```python
from build123d import *

# Parameters (mm, degrees)
BOSS_EXTRUDE1_DEPTH = 4.7
SKETCH2_R           = 8.5
BOSS_EXTRUDE2_DEPTH = 1
SKETCH4_R           = 6.5
SKETCH3_R           = 8.5
SKETCH5_R           = 4.25
BOSS_EXTRUDE3_DEPTH = 7
CHAMFER1_SIZE       = 0.4
SKETCH6_R           = 0.75
CUT_EXTRUDE1_DEPTH  = 7
CUT_EXTRUDE2_START  = -1
CUT_EXTRUDE2_DEPTH  = 1


with BuildPart() as part:
    # Sketch1 → Boss-Extrude1 (new body)
    with BuildSketch(Plane(origin=(0, 0, 0), x_dir=(1, 0, 0), z_dir=(0, 1, 0))):
        Polygon((0, 6.92820323), (6, 3.464101615), (6, -3.464101615), (0, -6.92820323), (-6, -3.464101615), (-6, 3.464101615), align=None)
    extrude(amount=BOSS_EXTRUDE1_DEPTH)

    # Sketch2 → Boss-Extrude2 (add)
    with BuildSketch(Plane(origin=(0, 4.7, 0), x_dir=(1, 0, 0), z_dir=(0, 1, 0))):
        with Locations(Location((0, 0, 0), (0, 0, 270))):
            Circle(SKETCH2_R)
    extrude(amount=BOSS_EXTRUDE2_DEPTH)

    # Sketch4 → Loft1 section 0
    with BuildSketch(Plane(origin=(0, 15.7, 0), x_dir=(1, 0, 0), z_dir=(0, 1, 0))):
        Circle(SKETCH4_R)
    # Sketch3 → Loft1 section 1
    with BuildSketch(Plane(origin=(0, 5.7, 0), x_dir=(1, 0, 0), z_dir=(0, 1, 0))):
        Circle(SKETCH3_R)
    loft()

    # Sketch5 → Boss-Extrude3 (add)
    with BuildSketch(Plane(origin=(0, 15.7, 0), x_dir=(1, 0, 0), z_dir=(0, 1, 0))):
        with Locations(Location((0, 0, 0), (0, 0, 270))):
            Circle(SKETCH5_R)
        with BuildLine():
            Line((-1.95, 2.044046232), (-1.95, -2.044046232))
            ThreePointArc((-1.95, -2.044046232), (0, -2.825), (1.95, -2.044046232))
            Line((1.95, -2.044046232), (1.95, 2.044046232))
            ThreePointArc((1.95, 2.044046232), (0, 2.825), (-1.95, 2.044046232))
        make_face(mode=Mode.SUBTRACT)
    extrude(amount=BOSS_EXTRUDE3_DEPTH)

    # Chamfer1
    chamfer1_edges = [part.edges().sort_by_distance(p)[0] for p in [
        (-6.5, 15.7, 0),
        (0, 22.7, -4.25),
        (0, 22.7, -2.825),
        (-1.95, 22.7, 0),
        (0, 22.7, 2.825),
        (1.95, 22.7, 0),
    ]]
    chamfer(chamfer1_edges, length=CHAMFER1_SIZE)

    # Sketch6 → Cut-Extrude1 (cut)
    with BuildSketch(Plane.XZ):
        with Locations(Location((0, 0, 0), (0, 0, 270))):
            Circle(SKETCH6_R)
    extrude(amount=-CUT_EXTRUDE1_DEPTH, mode=Mode.SUBTRACT)

    # Sketch7 → Cut-Extrude2 (cut)
    with BuildSketch(Plane(origin=(0, 15.7, 0), x_dir=(1, 0, 0), z_dir=(0, 1, 0)).offset(CUT_EXTRUDE2_START)):
        with BuildLine():
            Line((1.95, -2.044046232), (1.95, 2.044046232))
            ThreePointArc((1.95, 2.044046232), (0, 2.825), (-1.95, 2.044046232))
            Line((-1.95, 2.044046232), (-1.95, -2.044046232))
            ThreePointArc((-1.95, -2.044046232), (0, -2.825), (1.95, -2.044046232))
        make_face()
    extrude(amount=CUT_EXTRUDE2_DEPTH, mode=Mode.SUBTRACT)


solid = part.part
```
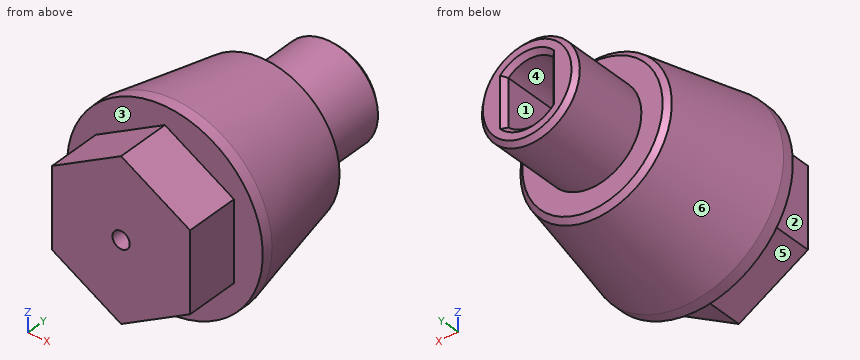
Can you work these out from the model? Positions are in its coordinate system, mm. Face numbers are marked on the shaded views. A direction names the side the tool comes from. Coordinates: 2 decimals unless noted, no trailing zeros. Loops run counter-clockwise (first coordinate to the right, second up) from the corner with the lowest first, then second, coordinate; pieces in that order, holes last.
1) Thinking about a two-plate mould opening in X: for the marked faces 4, 5 and 6, which applies, pulls with the +X half, pulls with the -X half, needs draft (parallel to the pull), parting line crosses it, or undercut?
2) Imagine slicing it at C-C on y = 6. List the corners of the cut face in (x, z) for me, plus the area to 3 significant figures.
3) For pin 1 (2 mm diameter, centred on x = 0, z = 0, fed in from +Y); pin 2 (5 mm diameter, centred on y = 3, z = 1, fed in from +X); pin 3 (3 mm diameter, centred on x = 0.5, z = -0.5, fed in from +Y); pin 4 (0.8 mm diameter, centred on x = 0, z = 0, fed in from -Y), each with a flat end and sliding along its axis, tell me the tip position at first contact or that it passes through.
4) Imagine slicing it at B-B on y = 13. List the corners of the cut face in (x, z) for me, plus the area to 3 significant figures.
5) Which directions (+Z, -Z, +X, -X, +Y, -Y) give clear straight access to the entire face, cutting with the end or side of a thin tool? Please do the marked faces 1, 2 and 3.
6) I need wall thicknesses on probe 1 along X at (y, z) = (3.75, 0); probe 2 along X at (y, z) = (5.5, 0); probe 3 along Y at (x, z) = (-4.5, 1.25). Which ranges of each line are inside material? Lowest first, please.
7) Imagine slicing it at A-A on y = 17.5. List the corners of the cut face in (x, z) for me (3 decimals), plus the area to 3 significant figures.
Completed:
1. face 4: undercut
1. face 5: pulls with the -X half
1. face 6: parting line crosses it
2. outline: circle Ø16.88 at (0, 0); hole circle Ø1.5 at (0, 0)
2. area: 222 mm2
3. pin 1: stops at y = 14.7
3. pin 2: stops at x = 8.5
3. pin 3: stops at y = 22.35
3. pin 4: stops at y = 7
4. outline: circle Ø14.08 at (0, 0)
4. area: 156 mm2
5. face 1: +Y
5. face 2: +Z, -Z, -X, -Y
5. face 3: -Y
6. probe 1: x = -6 to -0.75, 0.75 to 6
6. probe 2: x = -8.5 to -0.75, 0.75 to 8.5
6. probe 3: y = 0 to 15.7
7. outline: circle Ø8.5 at (0, 0); hole (-1.95, -2.044) arc R2.825 ccw to (1.95, -2.044) - (1.95, 2.044) arc R2.825 ccw to (-1.95, 2.044) - close
7. area: 36.6 mm2
